```python
from build123d import *

# Parameters (mm, degrees)
SKETCH1_R           = 1.89865
SKETCH1_R_2         = 1.4732
BOSS_EXTRUDE3_DEPTH = 6.0452
SKETCH7_R           = 1.4732
CUT_EXTRUDE2_DEPTH  = 93.2317735
SKETCH9_R           = 1.4732
SKETCH9_W           = 30.226
SKETCH9_H           = 47.117
CUT_EXTRUDE3_DEPTH  = 14.732
SKETCH10_R          = 2.54
SKETCH10_W          = 6.35
SKETCH10_H          = 3.175
SKETCH10_W_2        = 3.175
SKETCH10_H_2        = 6.35
CUT_EXTRUDE4_DEPTH  = 6.0452
SKETCH12_R          = 1.4732
CUT_EXTRUDE5_DEPTH  = 6.0452
SKETCH13_R          = 1.1684
CUT_EXTRUDE6_DEPTH  = 6.0452


with BuildPart() as part:
    # Sketch1 → Boss-Extrude3 (new body)
    with BuildSketch(Plane.XY):
        with BuildLine():
            Line((-53.34, 52.724229724), (-53.34, -52.724229724))
            ThreePointArc((-53.34, -52.724229724), (0, -75), (53.34, -52.724229724))
            Line((53.34, -52.724229724), (53.34, 52.724229724))
            ThreePointArc((53.34, 52.724229724), (43.863063402, 60.836104979), (33.172661219, 67.264957799))
            ThreePointArc((33.172661219, 67.264957799), (0, 47.904876359), (-33.172661219, 67.264957799))
            ThreePointArc((-33.172661219, 67.264957799), (-43.863063402, 60.836104979), (-53.34, 52.724229724))
        make_face()
        with Locations((0, -66.675)):
            Circle(SKETCH1_R, mode=Mode.SUBTRACT)
        with Locations((-44.45, 49.6966108)):
            Circle(SKETCH1_R, mode=Mode.SUBTRACT)
        with Locations(Location((44.45, 49.6966108, 0), (0, 0, 180))):
            Circle(SKETCH1_R, mode=Mode.SUBTRACT)
        with Locations((-21.59, -15.875)):
            Circle(SKETCH1_R_2, mode=Mode.SUBTRACT)
        with Locations((-6.35, -15.875)):
            Circle(SKETCH1_R_2, mode=Mode.SUBTRACT)
        with Locations(Location((6.35, -15.875, 0), (0, 0, 180))):
            Circle(SKETCH1_R_2, mode=Mode.SUBTRACT)
        with Locations((-15.24, -65.475)):
            Circle(SKETCH1_R_2, mode=Mode.SUBTRACT)
        with Locations(Location((15.24, -65.475, 0), (0, 0, 180))):
            Circle(SKETCH1_R_2, mode=Mode.SUBTRACT)
        with Locations(Location((21.59, -15.875, 0), (0, 0, 180))):
            Circle(SKETCH1_R_2, mode=Mode.SUBTRACT)
        with Locations((6.35, 15.875)):
            Circle(SKETCH1_R_2, mode=Mode.SUBTRACT)
        with Locations(Location((-6.35, 15.875, 0), (0, 0, 180))):
            Circle(SKETCH1_R_2, mode=Mode.SUBTRACT)
        with Locations((21.59, 15.875)):
            Circle(SKETCH1_R_2, mode=Mode.SUBTRACT)
        with Locations(Location((-21.59, 15.875, 0), (0, 0, 180))):
            Circle(SKETCH1_R_2, mode=Mode.SUBTRACT)
    extrude(amount=BOSS_EXTRUDE3_DEPTH)

    # Sketch7 → Cut-Extrude2 (cut, through all)
    with BuildSketch(Plane.XY.offset(6.0452)):
        with Locations(Location((-31.75, -41.98, 0), (0, 0, 180))):
            Circle(SKETCH7_R)
        with Locations((31.75, -41.98)):
            Circle(SKETCH7_R)
    extrude(amount=-CUT_EXTRUDE2_DEPTH, mode=Mode.SUBTRACT)

    # Sketch9 → Cut-Extrude3 (cut)
    with BuildSketch(Plane.XY.offset(6.0452)):
        with Locations((-16.51, 45.301376359)):
            Circle(SKETCH9_R)
        with Locations((16.51, 45.301376359)):
            Circle(SKETCH9_R)
        with Locations((-16.51, -9.308623641)):
            Circle(SKETCH9_R)
        with Locations((16.51, -9.308623641)):
            Circle(SKETCH9_R)
        with Locations((0, 17.996376359)):
            Rectangle(SKETCH9_W, SKETCH9_H)
    extrude(amount=-CUT_EXTRUDE3_DEPTH, mode=Mode.SUBTRACT)

    # Sketch10 → Cut-Extrude4 (cut)
    with BuildSketch(Plane.XY.offset(6.0452)):
        with Locations((-36.195, -44.469229724)):
            Circle(SKETCH10_R)
        with Locations((36.195, -44.469229724)):
            Circle(SKETCH10_R)
        with Locations((-38.1, 45.999876359)):
            Circle(SKETCH10_R)
        with Locations((38.1, 45.999876359)):
            Circle(SKETCH10_R)
        with Locations((-38.1, 58.699876359)):
            Rectangle(SKETCH10_W, SKETCH10_H)
        with Locations((38.1, 58.699876359)):
            Rectangle(SKETCH10_W, SKETCH10_H)
        with Locations((-43.815, -54.629229724)):
            Rectangle(SKETCH10_W_2, SKETCH10_H_2)
        with Locations((43.815, -54.629229724)):
            Rectangle(SKETCH10_W_2, SKETCH10_H_2)
    extrude(amount=-CUT_EXTRUDE4_DEPTH, mode=Mode.SUBTRACT)

    # Sketch12 → Cut-Extrude5 (cut)
    with BuildSketch(Plane.XY.offset(6.0452)):
        with Locations((22.733, 37.304304366)):
            Circle(SKETCH12_R)
        with Locations((30.790076227, 33.547228019)):
            Circle(SKETCH12_R)
        with Locations((38.847152454, 29.790151672)):
            Circle(SKETCH12_R)
        with Locations((46.90422868, 26.033075325)):
            Circle(SKETCH12_R)
        with Locations((22.733, 28.829624443)):
            Circle(SKETCH12_R)
        with Locations((29.543135099, 23.115242593)):
            Circle(SKETCH12_R)
        with Locations((36.353270199, 17.400860743)):
            Circle(SKETCH12_R)
        with Locations((43.163405298, 11.686478893)):
            Circle(SKETCH12_R)
        with Locations((-43.163405298, 11.686478893)):
            Circle(SKETCH12_R)
        with Locations((-36.353270199, 17.400860743)):
            Circle(SKETCH12_R)
        with Locations((-29.543135099, 23.115242593)):
            Circle(SKETCH12_R)
        with Locations((-22.733, 28.829624443)):
            Circle(SKETCH12_R)
        with Locations((-46.90422868, 26.033075325)):
            Circle(SKETCH12_R)
        with Locations((-38.847152454, 29.790151672)):
            Circle(SKETCH12_R)
        with Locations((-30.790076227, 33.547228019)):
            Circle(SKETCH12_R)
        with Locations((-22.733, 37.304304366)):
            Circle(SKETCH12_R)
    extrude(amount=-CUT_EXTRUDE5_DEPTH, mode=Mode.SUBTRACT)

    # Sketch13 → Cut-Extrude6 (cut)
    with BuildSketch(Plane.XY.offset(6.0452)):
        with Locations((22.832493661, 49.627795037)):
            Circle(SKETCH13_R)
        with Locations((-22.832493661, 49.627795037)):
            Circle(SKETCH13_R)
        with Locations((-28.455572264, 53.419074276)):
            Circle(SKETCH13_R)
        with Locations((28.455572264, 53.419074276)):
            Circle(SKETCH13_R)
    extrude(amount=-CUT_EXTRUDE6_DEPTH, mode=Mode.SUBTRACT)


solid = part.part
```
Part model, mm, in its own coordinate system. Round coordinates to 2 decimals unless told otherwise and drop trailing zeros. Loops run counter-clockwise (first coordinate to the right, second up) from the corner with the lowest first, then second, coordinate; pieces in that order, holes last.
Item 1: Mould opens along Y. For faces 1 (the face through (-1, -19, 6.045)), 2 (the face through (28.07, 23.18, 3.06)), 3 (the face through (-43.72, 60.94, 2.98)) say: +Y half, -Y half, draft (parallel to the pull), parting line (faces both ways), or undercut.
Item 2: Drill centre lines: line 1 (X direction, y = -9, z = 3.5); line 2 (X direction, y = 9.5, z = 0.5); line 3 (Y direction, x = -32, z = 5.25). Where is each one in solid material? Low to high.
Item 3: Drop flat-ended pins along their axis: P1, Ø4.5, axis at x = 36.35, y = 17.4, coming from the +Z side; P2, Ø1.6, axis at y = 58, z = 3, coming from the -X side; P3, Ø1, axis at x = 28, z = 3.5, coming from the +Y side; P4, Ø1.5, axis at x = 27.5, z = 1.5, coming from the +Y side. Give the stop position or say it passes through.
Item 4: Cut at B-B, the plane x = 0. Give the cut face in (y, z).
Item 5: Cut at C-C, the plane z = 4.25. State how many separate pieces and enclosed holes the cut face has, then the cut area to 3 significant figures.
Item 6: Cut at A-A, the plane y = 8.5. Give the cut face in (x, z).
A:
1. face 1: draft
1. face 2: undercut
1. face 3: +Y half
2. line 1: x = -53.34 to -17.95, -15.07 to 15.07, 17.95 to 53.34
2. line 2: x = -53.34 to -15.11, 15.11 to 53.34
2. line 3: y = -67.83 to -43.43, -40.53 to 32.71, 34.39 to 65.33
3. P1: stops at z = 6.05
3. P2: stops at x = -48.51
3. P3: stops at y = 60.72
3. P4: stops at y = 60.44
4. outline: (-75, 0) - (-68.57, 0) - (-68.57, 6.05) - (-75, 6.05) - close; (-64.78, 0) - (-5.56, 0) - (-5.56, 6.05) - (-64.78, 6.05) - close; (41.55, 0) - (47.9, 0) - (47.9, 6.05) - (41.55, 6.05) - close
5. separate pieces: 1
5. enclosed holes: 46
5. area: 11,400 mm2
6. outline: (-53.34, 0) - (-15.11, 0) - (-15.11, 6.05) - (-53.34, 6.05) - close; (15.11, 0) - (53.34, 0) - (53.34, 6.05) - (15.11, 6.05) - close
